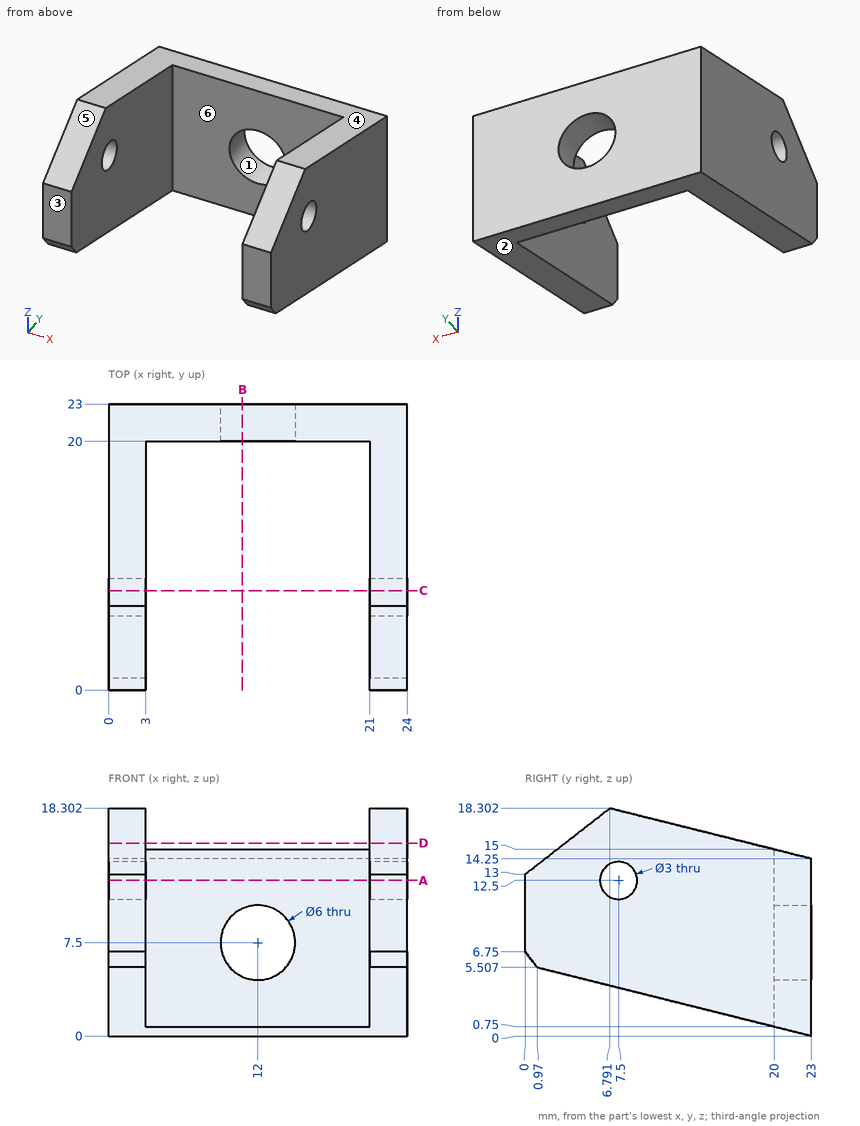
Check sheet for the drawn part. Datum: minimum x, y, z corner. Units: mm. A direction names the side the tool comes from. Round coordinates to 2 decimals unless told otherwise and drop trailing zeros. Order: outer loops, then holes, each group sorted by start corner. A loop starts at its lowest first (then second) coordinate and runs counter-clockwise, first axis right, second up.
(1) Scan lines: probe 1 along X at (y, z) = (18.5, 3.5); probe 2 along Y at (x, z) = (1.75, 12.5); probe 3 along Z at (x, y) = (22, 7.5) (1 decimal). Record each from-to range of solid material in increasing order.
(2) Go/stop test with flat-tipped pins: P1, Ø1.8, axis at y = 7.5, z = 12.5, coming from the -X side; P2, Ø10, axis at x = 10, z = 13, coming from the -Y side; P3, Ø6, axis at x = 2.5, y = 5, coming from the -Z side. Record where each tip stops, or that it passes through.
(3) Cross-section at C-C, the plane y = 8. State how many separate pieces and enclosed holes the cut face has.
(4) Draft check along Z on the marked faces 1, 2, 3 and 4. Enter one of: pulls with the +Z half, pulls with the -Z half, needs draft (parallel to the pull), parting line crosses it, or undercut.
(5) Cross-section at B-B, the plane x = 10.75. Enter the section's corners in (y, z), and give its area (3 significant figures).
(6) Cross-section at A-A, the plane z = 12.5. Enter the section's corners in (x, y), and give its area (3 significant figures).
(7) Access from +Z, -Z, +X, -X, +Y, -Y to the whole of each face (thin tool, end or side, straight path). Record for the marked faces 5 and 6.
(8) Cross-section at D-D, the plane z = 15.5. Enter the section's corners in (x, y).
Check sheet entries:
1. probe 1: x = 0 to 3, 21 to 24
1. probe 2: y = 0 to 6, 9 to 23
1. probe 3: z = 3.9 to 11, 14 to 18.1
2. P1: passes through
2. P2: stops at y = 20
2. P3: stops at z = 3.75
3. separate pieces: 4
3. enclosed holes: 0
4. face 1: undercut
4. face 2: pulls with the -Z half
4. face 3: needs draft
4. face 4: pulls with the +Z half
5. outline: (20, 0.75) - (23, 0) - (23, 4.77) - (20, 4.77) - close; (20, 10.23) - (23, 10.23) - (23, 14.25) - (20, 15) - close
5. area: 26.4 mm2
6. outline: (0, 0) - (3, 0) - (3, 6) - (0, 6) - close; (0, 9) - (3, 9) - (3, 20) - (21, 20) - (21, 9) - (24, 9) - (24, 23) - (0, 23) - close; (21, 0) - (24, 0) - (24, 6) - (21, 6) - close
6. area: 174 mm2
7. face 5: +Z, +X, -X, -Y
7. face 6: +Z, -Z, -Y
8. outline: (0, 3.2) - (3, 3.2) - (3, 18) - (0, 18) - close; (21, 3.2) - (24, 3.2) - (24, 18) - (21, 18) - close
